For this review, take the finished solid that the model builds, in its own axes (mm). A direction names the side the tool comes from. Give positions to 0.01 mm unless a question says otherwise; leave off trailing zeros. Order: outer loops, then holes, each group sorted by start corner. A loop starts at its lowest first (then second) coordinate and runs counter-clockwise, first axis right, second up. Notation, with made-up numbers: (61, 11) -> (83, 11) arc R9 ccw to (83, 20) -> close; hole circle Ø4 at (-35, 28.25). An arc over 180 degrees is marked (long way). Return JSON: item names as keys, results as strings. Group by question number.
1) Add section B-B (z = -15). Give the boundary of the cut face in (x, y), then the cut area to 3 significant figures.
2) For faces 4 (the face through (6.35, 16, -118)), 5 (the face through (3.22, 17.85, -208.57)), 6 (the face through (23.292, 3.846, -167.484)), list the 3-axis set-ups (+Z, -Z, +X, -X, +Y, -Y) from which the entire face can be reached by the end or side of a thin tool; tool diameter is ignored.
3) To check wall thickness, follow line 1 along Z through (x, y) = (3, 46.5); line 2 along X through (y, z) = (5, -70); line 3 along Z through (x, y) = (3.25, 22). State the ranges of each line that lie inside material, in increasing order.
4) The part is to be moulded in two halves that separate along X. For faces 1 (the face through (3, 16.35, -121)), 2 (the face through (24.283, 3.846, -71.944)), 3 (the face through (30, 3, -118)), say which applies: released by +X, released by -X, zero draft, split by the parting line, or undercut.
5) Add section A-A (y = 25). Give the boundary of the cut face in (x, z), then the cut area to 3 significant figures.
6) Add section C-C (y = 46.5). Give the boundary of the cut face in (x, z).
7) Add section D-D (z = -203). Give the boundary of the cut face in (x, y), then the cut area to 3 significant figures.
8) Insertion check: P1, Ø8, axis at y = 19.5, z = -82.5, coming from the +X side; P2, Ø6, axis at x = 21.5, z = -69, coming from the +Y side; P3, Ø3.5, axis at y = 46.5, z = -15, coming from the +X side; P4, Ø2.5, axis at x = 22.5, z = -171, coming from the +Y side. Each pin has a flat end and moves straight along its axis. Give the tip position at first contact, or say it passes through.
from build123d import *

# Parameters (mm, degrees)
EXTRUDE_THIN1_DEPTH                        = 240
SKETCH3_W                                  = 35
SKETCH3_H                                  = 300
EXTRUDE2_DEPTH                             = 7.35
SKETCH7_W                                  = 300
SKETCH7_H                                  = 30
EXTRUDE4_DEPTH                             = 7.35
EXTRUDE5_DEPTH                             = 7.35
TAPPED_HOLE_FOR_8_32_HELICOIL1_D           = 4.3942
TAPPED_HOLE_FOR_8_32_HELICOIL2_D           = 4.3942
TAPPED_HOLE_FOR_8_32_HELICOIL2_DEPTH       = 11.1252
TAPPED_HOLE_FOR_8_32_HELICOIL2_CBORE_D     = 5.27558
TAPPED_HOLE_FOR_8_32_HELICOIL2_CBORE_DEPTH = 5.08
TAPPED_HOLE_FOR_8_32_HELICOIL2_TIP         = 1.320150866
FILLET5_R                                  = 3


with BuildPart() as part:
    # Sketch1 → Extrude-Thin1 (new body)
    with BuildSketch(Plane.XY):
        Polygon((0, 55), (0, 0), (50.8, 0), (50.8, 6.35), (6.35, 6.35), (6.35, 55), align=None)
    extrude(amount=-EXTRUDE_THIN1_DEPTH)

    # Sketch3 → Extrude2 (cut, through all)
    with BuildSketch(Plane(origin=(0, 6.35, 0), x_dir=(1, 0, 0), z_dir=(0, 1, 0))):
        with Locations((47.5, 95)):
            Rectangle(SKETCH3_W, SKETCH3_H)
    extrude(amount=-EXTRUDE2_DEPTH, mode=Mode.SUBTRACT)

    # Sketch7 → Extrude4 (cut, through all)
    with BuildSketch(Plane(origin=(6.35, 0, 0), x_dir=(0, 0, -1), z_dir=(1, 0, 0))):
        with Locations((145, 67)):
            Rectangle(SKETCH7_W, SKETCH7_H)
    extrude(amount=-EXTRUDE4_DEPTH, mode=Mode.SUBTRACT)

    # Sketch10 → Extrude5 (cut, through all)
    with BuildSketch(Plane(origin=(6.35, 0, 0), x_dir=(0, 0, -1), z_dir=(1, 0, 0))):
        with BuildLine():
            Line((30, 66.35), (210, 66.35))
            Line((210, 66.35), (210, 21.35))
            ThreePointArc((210, 21.35), (208.535533906, 17.814466094), (205, 16.35))
            Line((205, 16.35), (35, 16.35))
            ThreePointArc((35, 16.35), (31.464466094, 17.814466094), (30, 21.35))
            Line((30, 21.35), (30, 66.35))
        make_face()
    extrude(amount=-EXTRUDE5_DEPTH, mode=Mode.SUBTRACT)

    # Tapped Hole for #8-32 Helicoil1 (through all)
    with Locations(Plane(origin=(6.35, 46.5, -15), x_dir=(0, 0, 1), z_dir=(1, 0, 0))):
        with Locations((0, 0), (-210, 0)):
            Hole(TAPPED_HOLE_FOR_8_32_HELICOIL1_D / 2)

    # Tapped Hole for #8-32 Helicoil2
    with Locations(Plane(origin=(22.5, 6.35, -70), x_dir=(0, 0, 1), z_dir=(0, 1, 0))):
        with Locations((0, 0), (-100, 0)):
            CounterBoreHole(TAPPED_HOLE_FOR_8_32_HELICOIL2_D / 2, TAPPED_HOLE_FOR_8_32_HELICOIL2_CBORE_D / 2, TAPPED_HOLE_FOR_8_32_HELICOIL2_CBORE_DEPTH, depth=TAPPED_HOLE_FOR_8_32_HELICOIL2_DEPTH)
            with Locations((0, 0, -(TAPPED_HOLE_FOR_8_32_HELICOIL2_DEPTH + TAPPED_HOLE_FOR_8_32_HELICOIL2_TIP / 2))):  # 118° drill point
                Cone(0, TAPPED_HOLE_FOR_8_32_HELICOIL2_D / 2, TAPPED_HOLE_FOR_8_32_HELICOIL2_TIP, mode=Mode.SUBTRACT)

    # Fillet5
    fillet5_edges = [part.edges().sort_by_distance(p)[0] for p in [
        (6.35, 6.35, -120),
        (0, 0, -120),
    ]]
    fillet(fillet5_edges, radius=FILLET5_R)


solid = part.part
Evaluation:
{
 "1": {"outline": "(0, 3) arc R3 ccw to (3, 0) -> (30, 0) -> (30, 6.35) -> (9.35, 6.35) arc R3 cw to (6.35, 9.35) -> (6.35, 44.3) -> (0, 44.3) -> close; (0, 48.7) -> (6.35, 48.7) -> (6.35, 52) -> (0, 52) -> close", "area": "452 mm^2"},
 "2": {"face 4": "+Z, -Z, +X, +Y", "face 5": "+X, -X, +Y", "face 6": "+Y"},
 "3": {"line 1": "-240 to -227.2, -222.8 to -210, -30 to -17.2, -12.8 to 0", "line 2": "0 to 19.86, 25.14 to 30", "line 3": "-240 to -210, -30 to 0"},
 "4": {"face 1": "zero draft", "face 2": "undercut", "face 3": "released by +X"},
 "5": {"outline": "(0, -240) -> (6.35, -240) -> (6.35, -210) -> (0, -210) -> close; (0, -30) -> (6.35, -30) -> (6.35, 0) -> (0, 0) -> close", "area": "381 mm^2"},
 "6": {"outline": "(0, -240) -> (6.35, -240) -> (6.35, -227.2) -> (0, -227.2) -> close; (0, -222.8) -> (6.35, -222.8) -> (6.35, -210) -> (0, -210) -> close; (0, -30) -> (6.35, -30) -> (6.35, -17.2) -> (0, -17.2) -> close; (0, -12.8) -> (6.35, -12.8) -> (6.35, 0) -> (0, 0) -> close"},
 "7": {"outline": "(0, 3) arc R3 ccw to (3, 0) -> (30, 0) -> (30, 6.35) -> (9.35, 6.35) arc R3 cw to (6.35, 9.35) -> (6.35, 16.35) -> (0, 16.35) -> close", "area": "254 mm^2"},
 "8": {"P1": "x = 6.35", "P2": "y = 6.35", "P3": "through", "P4": "y = 1.27"}
}
